```python
from build123d import *

# Parameters (mm, degrees)
SKETCH052_W     = 10
SKETCH052_H     = 10
PAD027_DEPTH    = 40
SKETCH053_R     = 1.3
POCKET002_DEPTH = 8
SKETCH054_R     = 1.3
POCKET003_DEPTH = 8


with BuildPart() as part:
    # Sketch052 → Pad027 (new body)
    with BuildSketch(Plane(origin=(0, 0, -60), x_dir=(1, 0, 0), z_dir=(0, 0, -1))):
        with Locations((-73, -10.5)):
            Rectangle(SKETCH052_W, SKETCH052_H)
    extrude(amount=-PAD027_DEPTH)

    # Sketch053 → Pocket002 (cut)
    with BuildSketch(Plane(origin=(0, 15.5, -60), x_dir=(1, 0, 0), z_dir=(0, 1, 0))):
        with Locations((-73, -5)):
            Circle(SKETCH053_R)
        with Locations((-73, -35)):
            Circle(SKETCH053_R)
    extrude(amount=-POCKET002_DEPTH, mode=Mode.SUBTRACT)

    # Sketch054 → Pocket003 (cut)
    with BuildSketch(Plane(origin=(-78, 0, -60), x_dir=(0, 1, 0), z_dir=(-1, 0, 0))):
        with Locations((10.5, -10)):
            Circle(SKETCH054_R)
        with Locations((10.5, -30)):
            Circle(SKETCH054_R)
    extrude(amount=-POCKET003_DEPTH, mode=Mode.SUBTRACT)


solid = part.part
```
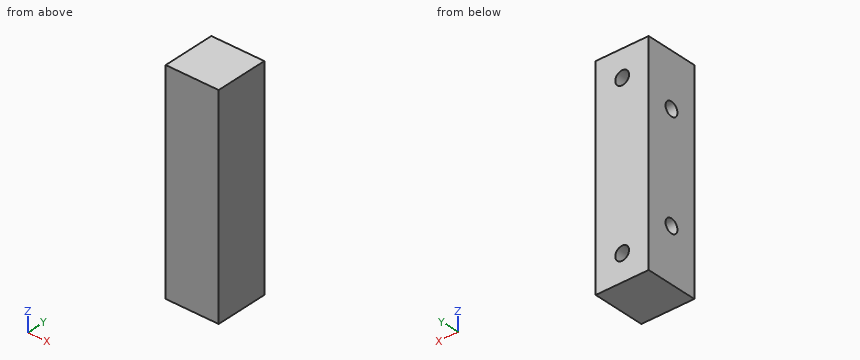
The model under review builds one solid part; all positions refer to its coordinate system, in mm. Round coordinates to 2 decimals unless told otherwise and drop trailing zeros. Write each loop counter-clockwise with the first axis right and the second up, starting at its lowest first coordinate (ties: lowest second). Pieces come first, ordered by that corner, then holes. Notation, with made-up numbers: (61, 86) -> (100, 86) arc R17 cw to (100, 101) -> close; hole circle Ø1 at (27.5, 42.25). An arc over 180 degrees is marked (long way). Use CSV: the item, a comma, the result in double quotes.
Q1. Consider section C-C (z = -50.5). Give the boundary of the cut face in (x, y).
Checks:
outline,"(-78, 5.5) -> (-68, 5.5) -> (-68, 15.5) -> (-78, 15.5) -> (-78, 11.7) -> (-70, 11.7) -> (-70, 9.3) -> (-78, 9.3) -> close"
Q2. To check wall thickness, follow probe 1 along Z at (x, y) = (-73, 9); probe 2 along Z at (x, y) = (-74.5, 10.5); probe 3 along X at (y, z) = (10.25, -55). State the ranges of each line that lie inside material, in increasing order. Write a range as [from, to].
Checks:
probe 1,"[-60, -56.3], [-53.7, -26.3], [-23.7, -20]"
probe 2,"[-60, -51.3], [-48.7, -31.3], [-28.7, -20]"
probe 3,"[-78, -74.3], [-71.7, -68]"
Q3. Consider section A-A (y = 10.5). Give the boundary of the cut face in (x, z), then the cut area to 3 significant figures.
Checks:
outline,"(-78, -60) -> (-68, -60) -> (-68, -20) -> (-78, -20) -> (-78, -28.7) -> (-70, -28.7) -> (-70, -31.3) -> (-78, -31.3) -> (-78, -48.7) -> (-70, -48.7) -> (-70, -51.3) -> (-78, -51.3) -> close; hole circle Ø2.6 at (-73, -55); hole circle Ø2.6 at (-73, -25)"
area,"348 mm²"
Q4. Consider section D-D (x = -73). Give the boundary of the cut face in (y, z), then the cut area to 3 significant figures.
Checks:
outline,"(5.5, -60) -> (15.5, -60) -> (15.5, -56.3) -> (7.5, -56.3) -> (7.5, -53.7) -> (15.5, -53.7) -> (15.5, -26.3) -> (7.5, -26.3) -> (7.5, -23.7) -> (15.5, -23.7) -> (15.5, -20) -> (5.5, -20) -> close; hole circle Ø2.6 at (10.5, -50); hole circle Ø2.6 at (10.5, -30)"
area,"348 mm²"
Q5. For pin 1 Ø0.8 at (y, z) = (10.5, -50) entering from -X; pin 2 Ø2.5 at (x, z) = (-73, -25) entering from +Y, all flat-tipped, find the tip position at first contact; note any pin that passes through.
Checks:
pin 1,"x = -70"
pin 2,"y = 7.5"
Q6. Consider section B-B (x = -75.75). Give the boundary of the cut face in (y, z), then the cut area to 3 significant figures.
Checks:
outline,"(5.5, -60) -> (15.5, -60) -> (15.5, -20) -> (5.5, -20) -> close; hole circle Ø2.6 at (10.5, -50); hole circle Ø2.6 at (10.5, -30)"
area,"389 mm²"
